For this review, take the finished solid that the model builds, in its own axes (mm). Face numbers are marked on the shaded views. Give positions to 0.01 mm unless a question says otherwise; leave off trailing zeros. Order: outer loops, then holes, each group sorted by start corner. A loop starts at its lowest first (then second) coordinate and runs counter-clockwise, first axis right, second up. Notation, with made-up numbers: M -15.5,89.5 L 21.5,89.5 A30 cw 21.5,118.5 Z; hole C -23.75,-40 d2. An arc over 180 degrees is marked long. Use CSV: the item, a comma, the result in double quotes. Start each with the question number.
(1) Consider section C-C (z = 23.5). Write out the cut boundary in (x, y), and give its area (3 significant figures).
(2) Wall thickness on L1, parallel to Z at x = -2.75, y = 4; L2, parallel to Y at x = -2.15, z = 35; L3, parallel to Z at x = -3.45, y = 21: over which ranges is each line inside the solid? List them lowest first. Write a range as from..to.
(3) Consider section D-D (z = 75.5). Write out the cut boundary in (x, y).
(4) Consider section B-B (y = 21). Write out the cut boundary in (x, z).
(5) Consider section A-A (x = -2.4). Write out the cut boundary in (y, z).
(6) Draft analysis for pull direction Z (two halves, no side actions). For the marked faces 1 and 2, state which applies: pulls with the +Z half, pulls with the -Z half, needs draft (parallel to the pull), parting line crosses it, or undercut.
(7) Clearance check with flat-ended pins moving along their axes: P1, Ø2.5, axis at x = -2, y = 1.5, coming from the -Z side; P2, Ø2, axis at x = -1.5, y = 23, coming from the +Z side; P3, Ø1, axis at x = -3, z = 28.5, coming from the -Y side. State where each tip first meets the part, or that it passes through.
```python
from build123d import *

# Parameters (mm, degrees)
F1_DEPTH = 5
F3_DEPTH = 5.001
F4_W     = 5
F4_H     = 10
F4_H_2   = 5
F4_H_3   = 67
F4_W_2   = 40
F4_W_3   = 10
F5_DEPTH = 5.001


with BuildPart() as f1:
    # F0 (on Right) → F1 (new body)
    with BuildSketch(Plane.YZ):
        Polygon((5, 97), (0, 97), (0, 0), (70, 0), (70, 5), align=None)
    extrude(amount=-F1_DEPTH)

    # F2 (on face) → F3 (cut, through all)
    with BuildSketch(Plane.YZ):
        with BuildLine():
            ThreePointArc((19.541804, 59.087683), (16.743201, 60.027803), (15, 57.645104))
            Line((15, 57.645104), (15, 17.5))
            ThreePointArc((15, 17.5), (15.732233, 15.732233), (17.5, 15))
            Line((17.5, 15), (45.863388, 15))
            ThreePointArc((45.863388, 15), (48.083349, 16.350315), (47.905193, 18.942579))
            Line((47.905193, 18.942579), (19.541804, 59.087683))
        make_face()
    extrude(amount=-F3_DEPTH, mode=Mode.SUBTRACT)

    # F4 (on face) → F5 (cut, through all)
    with BuildSketch(Plane.YZ):
        with Locations((2.5, 92)):
            Rectangle(F4_W, F4_H)
        with Locations((2.5, 79.5)):
            Rectangle(F4_W, F4_H_2)
        with Locations((2.5, 38.5)):
            Rectangle(F4_W, F4_H_3)
        with Locations((25, 2.5)):
            Rectangle(F4_W_2, F4_H_2)
        with Locations((2.5, 2.5)):
            Rectangle(F4_W, F4_H_2)
        with Locations((52.5, 2.5)):
            Rectangle(F4_W, F4_H_2)
        with Locations((65, 2.5)):
            Rectangle(F4_W_3, F4_H_2)
    extrude(amount=-F5_DEPTH, mode=Mode.SUBTRACT)


solid = f1.part
```
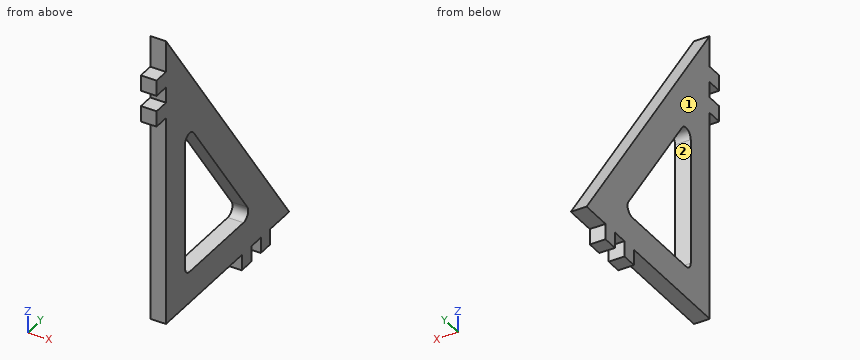
Check result:
1,outline,"M -5,5 L 0,5 L 0,15 L -5,15 Z; M -5,44.69 L 0,44.69 L 0,56.93 L -5,56.93 Z"
1,area,"111 mm^2"
2,L1,"z = 72..77, 82..87"
2,L2,"y = 5..15, 36.56..48.8"
2,L3,"z = 5..15, 57.02..74.35"
3,outline,"M -5,0 L 0,0 L 0,20.19 L -5,20.19 Z"
4,outline,"M -5,5 L 0,5 L 0,15 L -5,15 Z; M -5,57.02 L 0,57.02 L 0,74.35 L -5,74.35 Z"
5,outline,"M 0,72 L 5,72 L 5,5 L 45,5 L 45,0 L 50,0 L 50,5 L 55,5 L 55,0 L 60,0 L 60,5 L 70,5 L 5,97 L 5,87 L 0,87 L 0,82 L 5,82 L 5,77 L 0,77 Z; hole M 15,17.5 A2.5 ccw 17.5,15 L 45.86,15 A2.5 ccw 47.91,18.94 L 19.54,59.09 A2.5 ccw 15,57.65 Z"
6,face 1,"needs draft"
6,face 2,"undercut"
7,P1,"stops at z = 72"
7,P2,"stops at z = 72.94"
7,P3,"stops at y = 5"
